from build123d import *

# Parameters (mm, degrees)
ESQUISSE1_W             = 50
ESQUISSE1_H             = 25
BOSS_EXTRU_1_DEPTH      = 3
ESQUISSE2_R             = 3
BOSS_EXTRU_2_DEPTH      = 25
ESQUISSE3_R             = 2.5
ENL_V_MAT_EXTRU_1_DEPTH = 30.567718884


with BuildPart() as part:
    # Esquisse1 → Boss.-Extru.1 (new body)
    with BuildSketch(Plane.XY):
        Rectangle(ESQUISSE1_W, ESQUISSE1_H)
    extrude(amount=BOSS_EXTRU_1_DEPTH)

    # Esquisse2 → Boss.-Extru.2 (add, symmetric)
    with BuildSketch(Plane(origin=(0, 0, 0), x_dir=(0, 0, -1), z_dir=(1, 0, 0))):
        with Locations((-3, 12.5)):
            Circle(ESQUISSE2_R)
    extrude(amount=BOSS_EXTRU_2_DEPTH, both=True)

    # Esquisse3 → Enlèv. mat.-Extru.1 (cut, through all)
    with BuildSketch(Plane.XY.offset(3)):
        with Locations((-16, 0)):
            Circle(ESQUISSE3_R)
        with Locations((16, 0)):
            Circle(ESQUISSE3_R)
    extrude(amount=-ENL_V_MAT_EXTRU_1_DEPTH, mode=Mode.SUBTRACT)


solid = part.part
Input: part model. Units: mm. Frame: model coordinates. A direction names the side the tool comes from. Coordinates: 2 decimals unless noted, no trailing zeros. Loops run counter-clockwise (first coordinate to the right, second up) from the corner with the lowest first, then second, coordinate; pieces in that order, holes last. Notation, with made-up numbers: (24, 16.25) -> (37, 16.25) arc R23 ccw to (37, 49.25) -> close; hole circle Ø7 at (9, 86.5). An arc over 180 degrees is marked (long way). Write each question's results on one line, items separated by ' | '. Start each with the question number.
Q1. Reachability of faces 1 (the flat face through (0, 0, 0)), 2 (the flat face through (0, -1, 3)) from +Z, -Z, +X, -X, +Y, -Y: full face, straight path, thin tool, end or side. Return the list, or none.
Q2. Pull-direction query (Y, two-part tool) for faces 3 (the cylindrical face through (13.5, 0.1, 1.5)), 4 (the cylindrical face through (0.35, 14.69, 5.05)), 5 (the flat face through (-25, 5, 2)); classes: released by +Y, released by -Y, zero draft, split by the parting line, or undercut.
Q3. Section B-B, the plane x = 16. Return the cut outline in (y, z), plus the area to 3 significant figures.
Q4. Ray query, line 1 (Z direction, x = 8.5, y = -1.25); line 2 (Y direction, x = -15, z = 1); line 3 (Y direction, x = 16, z = 0.85). Return the intervals inside material, ascending. Write a range as from..to.
Q5. Section A-A, the plane y = 0. Return the cut outline in (x, z), plus the area to 3 significant figures.
Q6. Section C-C, the plane z = 0.7. Return the cut outline in (x, y).
Q7. Section D-D, the plane y = -5.75. Return the cut outline in (x, z), plus the area to 3 significant figures.
Q8. Pin query (flat end, axial travel): pin 1 (3 mm diameter, centred on x = -16, y = 0, fed in from +Z); pin 2 (12 mm diameter, centred on x = -1.5, y = -5.5, fed in from +Z). Return the tip coordinate at first contact, or that it passes through.
Found:
1) face 1: -Z, +X, -X, +Y, -Y | face 2: +Z, +X, -X, -Y
2) face 3: undercut | face 4: split by the parting line | face 5: zero draft
3) outline: (-12.5, 0) -> (-2.5, 0) -> (-2.5, 3) -> (-12.5, 3) -> close; (2.5, 0) -> (12.5, 0) arc R3 ccw (long way) to (9.5, 3) -> (2.5, 3) -> close | area: 81.2 mm2
4) line 1: 0..3 | line 2: -12.5..-2.29, 2.29..14.74 | line 3: -12.5..-2.5, 2.5..14.59
5) outline: (-25, 0) -> (-18.5, 0) -> (-18.5, 3) -> (-25, 3) -> close; (-13.5, 0) -> (13.5, 0) -> (13.5, 3) -> (-13.5, 3) -> close; (18.5, 0) -> (25, 0) -> (25, 3) -> (18.5, 3) -> close | area: 120 mm2
6) outline: (-25, -12.5) -> (25, -12.5) -> (25, 14.43) -> (-25, 14.43) -> close; hole circle Ø5 at (-16, 0); hole circle Ø5 at (16, 0)
7) outline: (-25, 0) -> (25, 0) -> (25, 3) -> (-25, 3) -> close | area: 150 mm2
8) pin 1: through | pin 2: z = 3
